Geometry: final body of the model. Coordinates: model frame, mm. Face numbers are marked on the shaded views. A direction names the side the tool comes from. Round coordinates to 2 decimals unless told otherwise and drop trailing zeros. Write each loop counter-clockwise with the first axis right and the second up, starting at its lowest first coordinate (ties: lowest second). Pieces come first, ordered by that corner, then holes.
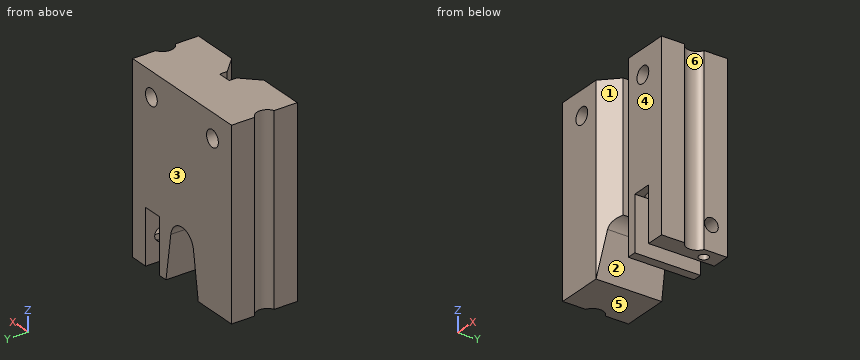
from build123d import *

# Parameters (mm, degrees)
F1_DEPTH = 54.7878
F2_R     = 2.4511
F2_W     = 5.715
F2_H     = 16.1798
F3_DEPTH = 25.4
F4_R     = 3.175
F5_DEPTH = 10.4648
F6_R     = 2.032
F7_DEPTH = 5.3975
F8_R     = 1.397
F9_DEPTH = 5.9421934451


with BuildPart() as f1:
    # F0 (on Top) → F1 (new body)
    with BuildSketch(Plane.XY):
        with BuildLine():
            Line((20.5486, 2.9099355663), (20.5486, 9.7536))
            Line((20.5486, 9.7536), (-20.5486, 9.7536))
            Line((-20.5486, 9.7536), (-20.5486, 2.918719736))
            ThreePointArc((-20.5486, 2.918719736), (-18.62328, 0), (-20.5486, -2.918719736))
            Line((-20.5486, -2.918719736), (-20.5486, -9.7536))
            Line((-20.5486, -9.7536), (-6.7096824712, -9.7536))
            Line((-6.7096824712, -9.7536), (-1.9939, -5.0378175288))
            Line((-1.9939, -5.0378175288), (-1.9939, -2.8194))
            Line((-1.9939, -2.8194), (1.9939, -2.8194))
            Line((1.9939, -2.8194), (1.9939, -5.0378175288))
            Line((1.9939, -5.0378175288), (6.7096824712, -9.7536))
            Line((6.7096824712, -9.7536), (20.5486, -9.7536))
            Line((20.5486, -9.7536), (20.5486, -2.9099355663))
            ThreePointArc((20.5486, -2.9099355663), (18.6436, 0), (20.5486, 2.9099355663))
        make_face()
    extrude(amount=F1_DEPTH)

    # F2 (on face) → F3 (cut)
    with BuildSketch(Plane.XZ.offset(9.7536)):
        with Locations((-12.6111, 47.5742)):
            Circle(F2_R)
        with Locations((12.7889, 47.5742)):
            Circle(F2_R)
        with Locations((12.2936, 8.0899)):
            Rectangle(F2_W, F2_H)
        with BuildLine():
            Line((6.7096824712, 0), (4.710379922, 13.4026572713))
            ThreePointArc((4.710379922, 13.4026572713), (0, 17.4625), (-4.710379922, 13.4026572713))
            Line((-4.710379922, 13.4026572713), (-6.7096824712, 0))
            Line((-6.7096824712, 0), (6.7096824712, 0))
        make_face()
    extrude(amount=-F3_DEPTH, mode=Mode.SUBTRACT)

    # F4 (on face) → F5 (cut)
    with BuildSketch(Plane(origin=(0, 0, 16.1798), x_dir=(1, 0, 0), z_dir=(0, 0, -1))):
        with Locations((11.4594824712, 4.318)):
            Circle(F4_R)
    extrude(amount=-F5_DEPTH, mode=Mode.SUBTRACT)

    # F6 (on face) → F7 (cut, through all)
    with BuildSketch(Plane.YZ.offset(20.5486)):
        with Locations((5.0546, 7.4168)):
            Circle(F6_R)
    extrude(amount=-F7_DEPTH, mode=Mode.SUBTRACT)

    # F8 (on face) → F9 (cut, through all)
    with BuildSketch(Plane(origin=(0, 0, 0), x_dir=(1, 0, 0), z_dir=(0, 0, -1))):
        with Locations((17.3736, -5.0546)):
            Circle(F8_R)
    extrude(amount=-F9_DEPTH, mode=Mode.SUBTRACT)


solid = f1.part
1) Section A-A on z = 40. Output: boundary loops of the cut face in (x, y) (3 decimals), plus the area to 3 significant figures.
2) Section D-D on x = 11.5. Output: boundary loops of the cut face in (y, z).
3) First-contact query: P1, Ø6.5, axis at x = -12.61, z = 47.57, coming from the +Y side; P2, Ø1.7, axis at x = 13.5, y = 3, coming from the -Z side; P3, Ø1.2, axis at x = 0, z = 34, coming from the -Y side; P4, Ø1.5, axis at y = -1, z = 14, coming from the +X side. Flat tips, straight axial feed; report the tip coordinate or a pass-through.
4) Draft query along Y for the marked faces 4, 5 and 6. Return one class per face: pulls with the +Y half, pulls with the -Y half, needs draft (parallel to the pull), parting line crosses it, or undercut.
5) Section B-B on z = 49. Output: boundary loops of the cut face in (x, y) (3 decimals), plus the area to 3 significant figures.
6) Line query: probe 1 along X at (y, z) = (-4.5, 4); probe 2 along X at (y, z) = (-8, 6); probe 3 along Z at (x, y) = (2, 3). Output: solid intervals per line, ascending.
7) Reachability of the marked faces 1, 2 and 3 from +Z, -Z, +X, -X, +Y, -Y: full face, straight path, thin tool, end or side. Return the list, or none.
8) Section C-C on y = 2.25. Output: boundary loops of the cut face in (x, z) (1 decimal), plus the area to 3 significant figures.
Filled in:
1. outline: (-20.549, -9.754) - (-6.71, -9.754) - (-1.994, -5.038) - (-1.994, -2.819) - (1.994, -2.819) - (1.994, -5.038) - (6.71, -9.754) - (20.549, -9.754) - (20.549, -2.91) arc R3.175 cw to (20.549, 2.91) - (20.549, 9.754) - (-20.549, 9.754) - (-20.549, 2.919) arc R3.175 cw to (-20.549, -2.919) - close
1. area: 736 mm2
2. outline: (-9.75, 16.18) - (-7.49, 16.18) - (-7.49, 26.64) - (-1.14, 26.64) - (-1.14, 16.18) - (9.75, 16.18) - (9.75, 45.49) - (-9.75, 45.49) - close; (-9.75, 49.66) - (9.75, 49.66) - (9.75, 54.79) - (-9.75, 54.79) - close
3. P1: stops at y = 9.75
3. P2: stops at z = 16.18
3. P3: stops at y = -2.82
3. P4: stops at x = 19.17
4. face 4: pulls with the -Y half
4. face 5: needs draft
4. face 6: undercut
5. outline: (-20.549, -9.754) - (-14.605, -9.754) - (-14.605, 9.754) - (-20.549, 9.754) - (-20.549, 2.919) arc R3.175 cw to (-20.549, -2.919) - close; (-10.617, -9.754) - (-6.71, -9.754) - (-1.994, -5.038) - (-1.994, -2.819) - (1.994, -2.819) - (1.994, -5.038) - (6.71, -9.754) - (10.795, -9.754) - (10.795, 9.754) - (-10.617, 9.754) - close; (14.783, -9.754) - (20.549, -9.754) - (20.549, -2.91) arc R3.175 cw to (20.549, 2.91) - (20.549, 9.754) - (14.783, 9.754) - close
5. area: 580 mm2
6. probe 1: x = -20.55 to -6.11, 6.11 to 9.44, 15.15 to 20.55
6. probe 2: x = -20.55 to -5.81, 5.81 to 9.44, 15.15 to 20.55
6. probe 3: z = 17.02 to 54.79
7. face 1: +Z, -Z, -Y
7. face 2: -Z, +Y, -Y
7. face 3: +Z, -Z, +X, -X, +Y
8. outline: (-19.6, 0) - (-6.7, 0) - (-4.7, 13.4) arc R4.8 cw to (4.7, 13.4) - (6.7, 0) - (9.4, 0) - (9.4, 16.2) - (15.2, 16.2) - (15.2, 0) - (19.6, 0) - (19.6, 54.8) - (-19.6, 54.8) - close; hole circle Ø4.9 at (-12.6, 47.6); hole circle Ø4.9 at (12.8, 47.6)
8. area: 1,830 mm2
